Read the model definition and answer for the solid it produces. Units are mm, in the model's axes. Face numbers are marked on the shaded views. Give positions to 0.01 mm unless a question says otherwise; leave off trailing zeros. Loops run counter-clockwise (first coordinate to the right, second up) from the corner with the lowest first, then second, coordinate; pieces in that order, holes last. Notation, with made-up numbers: (9.5, 19.25) -> (63.5, 19.25) arc R12 ccw to (63.5, 39.25) -> close; hole circle Ø5 at (82, 42). An arc over 180 degrees is marked (long way). Answer as CSV lines item,"result". Start each with the question number.
```python
from build123d import *

# Parameters (mm, degrees)
SKETCH1_W           = 249.6
SKETCH1_H           = 284.42
SKETCH1_R           = 2.5
SKETCH1_W_2         = 33
SKETCH1_H_2         = 90
BOSS_EXTRUDE1_DEPTH = 5
SKETCH4_W           = 133
SKETCH4_H           = 244.46665057
CUT_EXTRUDE2_DEPTH  = 49.034766894
CUT_EXTRUDE3_DEPTH  = 6
CUT_EXTRUDE4_DEPTH  = 6
SKETCH7_W           = 5
SKETCH7_H           = 20
SKETCH7_H_2         = 25
CUT_EXTRUDE5_DEPTH  = 6


with BuildPart() as part:
    # Sketch1 → Boss-Extrude1 (new body)
    with BuildSketch(Plane.XY):
        with Locations((124.8, -142.21)):
            Rectangle(SKETCH1_W, SKETCH1_H)
        with Locations((245.6, -26.5)):
            Circle(SKETCH1_R, mode=Mode.SUBTRACT)
        with Locations((245.6, -77.5)):
            Circle(SKETCH1_R, mode=Mode.SUBTRACT)
        with Locations((4, -77.5)):
            Circle(SKETCH1_R, mode=Mode.SUBTRACT)
        with Locations((4, -26.5)):
            Circle(SKETCH1_R, mode=Mode.SUBTRACT)
        with Locations((201.66, -52)):
            Rectangle(SKETCH1_W_2, SKETCH1_H_2, mode=Mode.SUBTRACT)
        with Locations((47.94, -52)):
            Rectangle(SKETCH1_W_2, SKETCH1_H_2, mode=Mode.SUBTRACT)
    extrude(amount=BOSS_EXTRUDE1_DEPTH)

    # Sketch4 → Cut-Extrude2 (cut, through all)
    with BuildSketch(Plane(origin=(0, -141.18753923, 110.307795042), x_dir=(1, 0, 0), z_dir=(0, 0.788010754, -0.615661475))):
        with Locations((68.5, 84.166930672)):
            Rectangle(SKETCH4_W, SKETCH4_H)
    extrude(amount=-CUT_EXTRUDE2_DEPTH, mode=Mode.SUBTRACT)

    # Sketch5 → Cut-Extrude3 (cut, through all)
    with BuildSketch(Plane.XY.offset(5)):
        Polygon((76.149175745, -159.084342324), (158.149444505, -51.841832454), (328.08312673, -181.777318211), (207.31876811, -339.716714228), (135, -284.42), (135, -200.788988557), align=None)
    extrude(amount=-CUT_EXTRUDE3_DEPTH, mode=Mode.SUBTRACT)

    # Sketch6 → Cut-Extrude4 (cut, through all)
    with BuildSketch(Plane.XY.offset(5)):
        Polygon((0, -94.564658056), (67.52306177, -146.194456905), (40.18963885, -181.941960195), (-27.33342292, -130.312161346), align=None)
    extrude(amount=-CUT_EXTRUDE4_DEPTH, mode=Mode.SUBTRACT)

    # Sketch7 → Cut-Extrude5 (cut, through all)
    with BuildSketch(Plane.XY.offset(5)):
        with Locations((17.788155616, -47.477871486)):
            Rectangle(SKETCH7_W, SKETCH7_H)
        with Locations((231.811844384, -47.477871486)):
            Rectangle(SKETCH7_W, SKETCH7_H)
        with Locations((17.788155616, -89.977871486)):
            Rectangle(SKETCH7_W, SKETCH7_H_2)
        with Locations((231.811844384, -89.977871486)):
            Rectangle(SKETCH7_W, SKETCH7_H_2)
    extrude(amount=-CUT_EXTRUDE5_DEPTH, mode=Mode.SUBTRACT)


solid = part.part
```
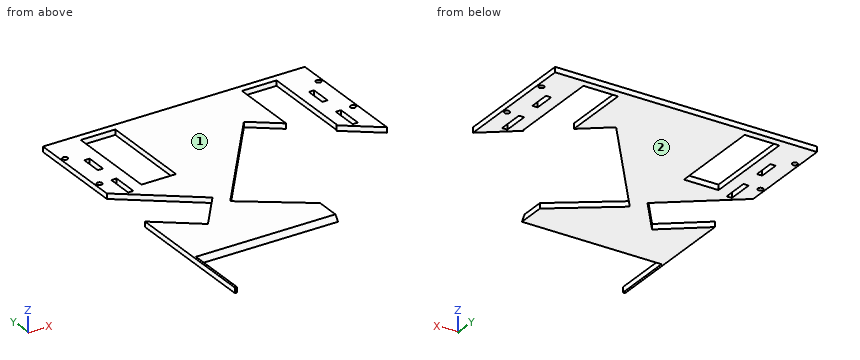
(1) Each of these flat-tipped pins is pushed along its axis until it touches: P1, Ø3, axis at x = 245.6, y = -26.5, coming from the +Z side; P2, Ø2.5, axis at y = -209.5, z = 2.5, coming from the +X side; P3, Ø1.5, axis at x = 54, z = 2, coming from the -Y side; P4, Ø1.5, axis at y = -123, z = 4, coming from the -X side. Where does it stop, or does it pass through?
(2) Find section D-D on z = 2.05. Give the number of separate pieces and of enclosed holes in the cut face, then the cut area to 3 significant figures.
(3) Find section B-B on x = 122.5. Write down the section's boundary in (y, z).
(4) Find the intervals of material crossed by line 1 along X through (y, z) = (-37, 4.5); line 2 along Y through (x, z) = (57, 2.6); line 3 along Y through (x, z) = (4, 3.05), in increasing order. Write a range as from..to.
(5) Find section A-A on y = -43. Write down the section's boundary in (x, z).
(6) Find section C-C on x = 60. Write down the section's boundary in (y, z), then the cut area to 3 significant figures.
(7) The mould has two halves that part along Z. Classify the marked faces 1 and 2: pulls with the +Z half, pulls with the -Z half, needs draft (parallel to the pull), parting line crosses it, or undercut.
Answer block:
1,P1,"passes through"
1,P2,"stops at x = 135"
1,P3,"stops at y = -226.39"
1,P4,"stops at x = 36.21"
2,separate pieces,"1"
2,enclosed holes,"9"
2,area,"27,500 mm2"
3,outline,"(-227.37, 0) -> (-191.93, 0) -> (-191.93, 5) -> (-223.46, 5) -> close; (-98.47, 0) -> (0, 0) -> (0, 5) -> (-98.47, 5) -> close"
4,line 1,"x = 0..31.44, 64.44..185.16, 218.16..249.6"
4,line 2,"y = -225.34..-159.96, -138.15..-97, -7..0"
4,line 3,"y = -224.99..-154.27, -97.62..-80, -75..-29, -24..0"
5,outline,"(0, 0) -> (15.29, 0) -> (15.29, 5) -> (0, 5) -> close; (20.29, 0) -> (31.44, 0) -> (31.44, 5) -> (20.29, 5) -> close; (64.44, 0) -> (185.16, 0) -> (185.16, 5) -> (64.44, 5) -> close; (218.16, 0) -> (229.31, 0) -> (229.31, 5) -> (218.16, 5) -> close; (234.31, 0) -> (249.6, 0) -> (249.6, 5) -> (234.31, 5) -> close"
6,outline,"(-227.37, 0) -> (-156.03, 0) -> (-156.03, 5) -> (-223.46, 5) -> close; (-140.44, 0) -> (-97, 0) -> (-97, 5) -> (-140.44, 5) -> close; (-7, 0) -> (0, 0) -> (0, 5) -> (-7, 5) -> close"
6,area,"599 mm2"
7,face 1,"pulls with the +Z half"
7,face 2,"pulls with the -Z half"
